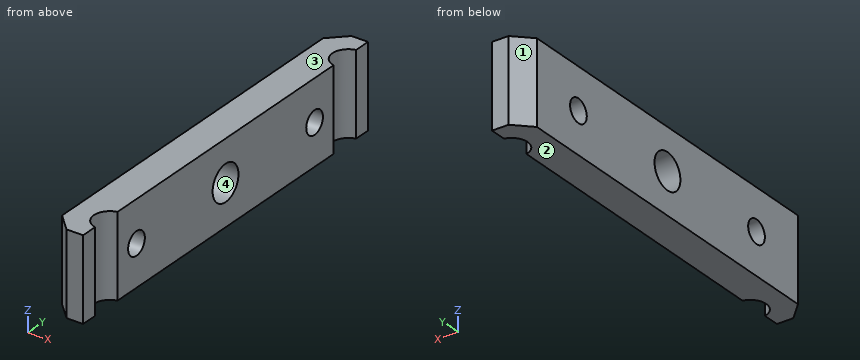
Autodesk Inventor part; units mm, degrees
ref_plane "YZ Plane" through (0, 0, 0) normal (1, 0, 0) x (0, 1, 0)
ref_plane "XZ Plane" through (0, 0, 0) normal (0, 1, 0) x (-1, 0, 0)
ref_plane "XY Plane" through (0, 0, 0) normal (0, 0, 1) x (1, 0, 0)
sketch "Szkic1" plane through (0, 0, 0) normal (0, 0, 1) x (1, 0, 0)
  circle A0 centre (0, 30) radius 3 construction
  arc A1 (-0.6454, 32.8273) -> (-0.6454, 27.1727) centre (0, 30) ccw
  line L0 (-0.6454, 27.1727) -> (-0.6454, 0)
  line L1 (-0.6454, 32.8273) -> (-0.6454, 35.8273)
  line L2 (-0.6454, 35.8273) -> (-3.6454, 35.8273)
  line L3 (-3.6454, 35.8273) -> (-6.6454, 32.8273)
  line L4 (-6.6454, 32.8273) -> (-6.6454, 0)
  line L5 (-0.6454, 0) -> (-6.6454, 0)
  point P0 (0, 0)
  dimension "d0" = 6
  dimension "d1" = 30
  dimension "d2" = 5.8
  dimension "d3" = 3
  dimension "d4" = 45
  dimension "d5" = 3
  dimension "d6" = 3
extrude "Wyciągnięcie proste1" add sketch "Szkic1" along normal blind 15
sketch "Szkic2" plane through (-6.6454, 0, 0) normal (-1, 0, 0) x (0, 0, 1)
  circle A0 centre (7.5, 22.3961) radius 2.1
  line L0 (0, 32.8273) -> (15, 32.8273)
  point P0 (0, 0)
  point P1 (7.5, 32.8273)
  dimension "d9" = 4.2
extrude "Wyciągnięcie proste2" cut sketch "Szkic2" against normal blind 8
mirror "Odbij1" about plane through (-6.6454, 0, 0) normal (0, -1, 0) of "Wyciągnięcie proste1", "Wyciągnięcie proste2"
sketch "Szkic3" plane through (-6.6454, 32.8273, 0) normal (-1, 0, 0) x (0, 0, 1)
  circle A0 centre (7.5, -32.8273) radius 3.25
  line L0 (0, 3) -> (15, 3)
  line L1 (0, 0) -> (0, -65.6545)
  point P0 (0, -32.8273)
  point P1 (7.5, 3)
  point P2 (0, -32.8273)
  point P3 (0, -32.8273)
  dimension "d12" = 6.5
extrude "Wyciągnięcie proste3" cut sketch "Szkic3" against normal through all
properties part number "6xMounting_clamp"
Input: part model. Units: mm. Frame: model coordinates. Face numbers are marked on the shaded views. Give positions to 0.01 mm unless a question says otherwise; leave off trailing zeros. Order: outer loops, then holes, each group sorted by start corner. A loop starts at its lowest first (then second) coordinate and runs counter-clockwise, first axis right, second up. Notation, with made-up numbers: (-34, 80) - (-4, 80) arc R17 ccw to (-4, 96) - close; hole circle Ø4 at (52.5, -31). An arc over 180 degrees is marked (long way). Write each question's results on one line, items separated by ' | '.
Item 1: Contact query for flat-ended pins moving along their axis: pin 1 Ø1.5 at (x, z) = (-4.5, 10.5) entering from -Y; pin 2 Ø2 at (x, z) = (-5.5, 11.5) entering from +Y. Output: stop coordinate, or through.
A:
pin 1: stops at y = -35.72 | pin 2: stops at y = 34.97
Item 2: Section B-B (y = 0). Return loops of the section in (x, z), and give its area (3 significant figures).
A:
outline: (-6.65, 0) - (-0.65, 0) - (-0.65, 4.25) - (-6.65, 4.25) - close; (-6.65, 10.75) - (-0.65, 10.75) - (-0.65, 15) - (-6.65, 15) - close | area: 51.0 mm^2
Item 3: Section A-A (z = 7.5). Return loops of the section in (x, y).
A:
outline: (-6.65, -32.83) - (-3.65, -35.83) - (-0.65, -35.83) - (-0.65, -32.83) arc R2.9 cw to (-0.65, -27.17) - (-0.65, -24.5) - (-6.65, -24.5) - close; (-6.65, -20.3) - (-0.65, -20.3) - (-0.65, -3.25) - (-6.65, -3.25) - close; (-6.65, 3.25) - (-0.65, 3.25) - (-0.65, 20.3) - (-6.65, 20.3) - close; (-6.65, 24.5) - (-0.65, 24.5) - (-0.65, 27.17) arc R2.9 cw to (-0.65, 32.83) - (-0.65, 35.83) - (-3.65, 35.83) - (-6.65, 32.83) - close
Item 4: Draft query along Z for the marked faces 1, 2, 3 and 4. Return one class per face: released by +Z, released by -Z, zero draft, split by the parting line, or undercut.
A:
face 1: zero draft | face 2: released by -Z | face 3: released by +Z | face 4: undercut
Item 5: Section D-D (z = 14.25). Return loops of the section in (x, y).
A:
outline: (-6.65, -32.83) - (-3.65, -35.83) - (-0.65, -35.83) - (-0.65, -32.83) arc R2.9 cw to (-0.65, -27.17) - (-0.65, 27.17) arc R2.9 cw to (-0.65, 32.83) - (-0.65, 35.83) - (-3.65, 35.83) - (-6.65, 32.83) - close
Item 6: Section C-C (x = -5.85). Return loops of the section in (y, z).
A:
outline: (-33.62, 0) - (33.62, 0) - (33.62, 15) - (-33.62, 15) - close; hole circle Ø4.2 at (-22.4, 7.5); hole circle Ø6.5 at (0, 7.5); hole circle Ø4.2 at (22.4, 7.5)
Item 7: Material intervals for line 1 along Y through (x, z) = (-3.5, 7.5); line 2 along Y through (x, z) = (-2.35, 7.5); line 3 along Y through (x, z) = (-1.1, 14.75), sorted ascending.
A:
line 1: y = -35.83 to -24.5, -20.3 to -3.25, 3.25 to 20.3, 24.5 to 35.83 | line 2: y = -35.83 to -31.7, -28.3 to -24.5, -20.3 to -3.25, 3.25 to 20.3, 24.5 to 28.3, 31.7 to 35.83 | line 3: y = -35.83 to -32.68, -27.32 to 27.32, 32.68 to 35.83
